```python
from build123d import *

# Parameters (mm, degrees)
CUT_EXTRUDE2_DEPTH      = 125.51506435
CUT_EXTRUDE2_DEPTH_BACK = 125.51506435
SKETCH7_W               = 25.4
SKETCH7_H               = 50.8
CUT_EXTRUDE3_DEPTH      = 254


with BuildPart() as part:
    # Sketch1 → Revolve1 (revolve)
    with BuildSketch(Plane.XY, mode=Mode.PRIVATE) as revolve1_sk:
        with BuildLine():
            Line((0, 0), (34.925, 0))
            Line((34.925, 0), (25.4, 25.4))
            Line((25.4, 25.4), (25.4, 107.494090512))
            ThreePointArc((25.4, 107.494090512), (13.148007491, 112.569031975), (0, 114.3))
            Line((0, 114.3), (0, 0))
        make_face()
    revolve(revolve1_sk.sketch.rotate(Axis((0, 114.3, 0), (0, -1, 0)), 90), axis=Axis((0, 114.3, 0), (0, -1, 0)))

    # Sketch6 → Cut-Extrude2 (cut, two sides: drawn at the far end of the back side and taken through both)
    with BuildSketch(Plane.XY.offset(-CUT_EXTRUDE2_DEPTH_BACK)):
        Polygon((-15.875, 56.694090512), (-25.4, 25.4), (-28.70874161, 28.70874161), (-29.778723272, 127.895690519), (-15.875, 127.895690519), align=None)
        Polygon((15.875, 127.895690519), (29.778723272, 127.895690519), (28.70874161, 28.70874161), (25.4, 25.4), (15.875, 56.694090512), align=None)
    extrude(amount=CUT_EXTRUDE2_DEPTH + CUT_EXTRUDE2_DEPTH_BACK, mode=Mode.SUBTRACT)

    # Sketch7 → Cut-Extrude3 (cut)
    with BuildSketch(Plane(origin=(15.875, 0, 0), x_dir=(0, 0, -1), z_dir=(1, 0, 0))):
        with Locations((0, 82.094090512)):
            Rectangle(SKETCH7_W, SKETCH7_H)
    extrude(amount=-CUT_EXTRUDE3_DEPTH, mode=Mode.SUBTRACT)


solid = part.part
```
Design review of the part built by this model. Coordinates are the model's own, in mm. A direction names the side the tool comes from. Coordinates: 2 decimals unless noted, no trailing zeros. Order: outer loops, then holes, each group sorted by start corner. A loop starts at its lowest first (then second) coordinate and runs counter-clockwise, first axis right, second up.
1) Mouldability with a two-part tool opening along Z and no side actions: class faces 1 (the flat face through (-19.512, 44.743, -0.278)), 2 (the flat face through (0, 107.494, 0)), 3 (the cylindrical face through (0.559, 57.9, 25.394)), 4 (the cylindrical face through (-0.559, 57.9, -25.394)) as +Z half, -Z half, draft (parallel to the pull), parting line (faces both ways), or undercut.
2) Clearance check with flat-ended pins moving along their axes: pin 1 (3 mm diameter, centred on y = 79.5, z = 15, fed in from -X) (3 decimals); pin 2 (1 mm diameter, centred on y = 18, z = -14.5, fed in from +X); pin 3 (1 mm diameter, centred on x = 20, y = 15, fed in from +Z). State where each tip first meets the part, or that it passes through.
3) Wall thickness on line 1 along X through (y, z) = (59, -17) (3 decimals); line 2 along Y through (x, z) = (4.5, 10.5); line 3 along Z through (x, y) = (-14, 93): over which ranges is each line inside the solid? List them lowest first.
4) Take a section at A-A, the plane y = 73.5. Give the boundary of the cut face in (x, z) (3 decimals), and give its area (3 significant figures).
5) For faces 5 (the flat face through (0, 82, 12.7)), 6 (the flat face through (15.875, 84, -13)), 7 (the flat face through (0, 0, 0)), 8 (the flat face through (-15.875, 85, 13)), 9 (the conical face through (-7.768, 24.167, 24.668)), list the 3-axis set-ups (+Z, -Z, +X, -X, +Y, -Y) from which the entire face can be reached by the end or side of a thin tool; tool diameter is ignored.
6) Take a section at D-D, the plane y = 9.5. Give the boundary of the cut face in (x, z) (1 decimal).
7) Take a section at C-C, the plane y = 53.5. Give the boundary of the cut face in (x, z), and give its area (3 significant figures).
8) Take a section at B-B, the plane x = 0. Give the boundary of the cut face in (y, z) (3 decimals).
Returned:
1. face 1: draft
1. face 2: undercut
1. face 3: +Z half
1. face 4: -Z half
2. pin 1: stops at x = -15.875
2. pin 2: stops at x = 24.52
2. pin 3: stops at z = 21.93
3. line 1: x = -15.875 to 15.875
3. line 2: y = 0 to 56.69, 107.49 to 113
3. line 3: z = -21.19 to -12.7, 12.7 to 21.19
4. outline: (-15.875, -19.828) arc R25.4 ccw to (15.875, -19.828) - (15.875, -12.7) - (-15.875, -12.7) - close; (-15.875, 12.7) - (15.875, 12.7) - (15.875, 19.828) arc R25.4 ccw to (-15.875, 19.828) - close
4. area: 694 mm2
5. face 5: +X, -X
5. face 6: +Z, -Z, +X, +Y
5. face 7: +Z, -Z, +X, -X, -Y
5. face 8: +Z, -Z, -X, +Y
5. face 9: +Y
6. outline: circle Ø62.7 at (0, 0)
7. outline: (-16.85, -19.01) arc R25.4 ccw to (16.85, -19.01) - (16.85, 19.01) arc R25.4 ccw to (-16.85, 19.01) - close
7. area: 1,580 mm2
8. outline: (0, -34.925) - (25.4, -25.4) - (107.494, -25.4) arc R50.8 ccw to (107.494, 25.4) - (25.4, 25.4) - (0, 34.925) - close; hole (56.694, -12.7) - (107.494, -12.7) - (107.494, 12.7) - (56.694, 12.7) - close
